CAD build for the part. Positions are in the model's coordinates, mm. Face numbers are marked on the shaded views. A direction names the side the tool comes from. Give positions to 0.01 mm unless a question says otherwise; leave off trailing zeros. Loops run counter-clockwise (first coordinate to the right, second up) from the corner with the lowest first, then second, coordinate; pieces in that order, holes last.
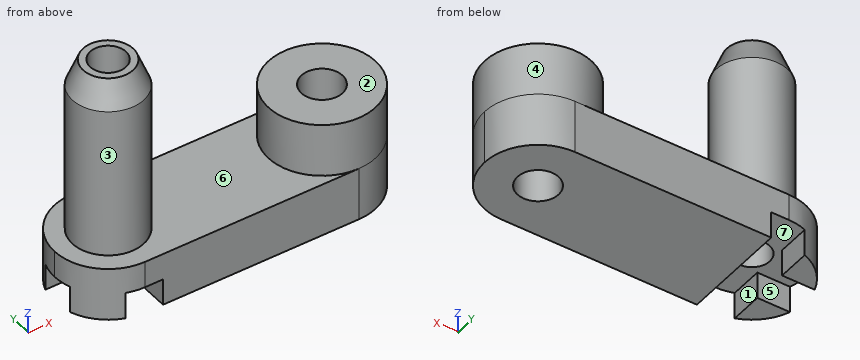
```python
from build123d import *

# Parameters (mm, degrees)
F0_W      = 18
F0_H      = 6
F1_DEPTH  = 3
F2_R      = 3
F2_R_2    = 2
F3_DEPTH  = 10
F4_R      = 1
F4_R_2    = 1.15
F5_DEPTH  = 20
F6_SIZE2  = 1.5
F6_SIZE   = 0.6
F7_W      = 11.6012076614
F7_H      = 11.8295210414
F8_DEPTH  = 7
F9_R      = 2.9999
F10_W     = 5.4413094251
F10_H     = 2
F11_DEPTH = 1.5


# Not quite as in the source:
# - a fillet or chamfer is up to 0.001 mm smaller than in the source, because OpenCascade refuses the exact size


with BuildPart() as f1:
    # F0 (on Top) → F1 (new body)
    with BuildSketch(Plane.XY):
        with Locations((1.8924829921, 0)):
            Rectangle(F0_W, F0_H)
    extrude(amount=F1_DEPTH)

    # F2 (on face) → F3 (join)
    with BuildSketch(Plane.XY.offset(3)):
        with Locations((7.8924829921, 0)):
            Circle(F2_R)
        with Locations((-4.1075170079, 0)):
            Circle(F2_R_2)
    extrude(amount=F3_DEPTH)

    # F4 (on face) → F5 (cut)
    with BuildSketch(Plane.XY.offset(13)):
        with Locations((-4.1075170079, 0)):
            Circle(F4_R)
        with Locations((7.8924829921, 0)):
            Circle(F4_R_2)
    extrude(amount=-F5_DEPTH, mode=Mode.SUBTRACT)

    # F6
    f6_edges = [f1.edges().sort_by_distance(p)[0] for p in [
        (-6.107517, 0, 13),
    ]]
    f6_side = f1.faces().sort_by_distance((-6.050948, 0, 13))[0]
    chamfer(f6_edges, length=F6_SIZE, length2=F6_SIZE2, reference=f6_side)

    # F7 (on face) → F8 (cut)
    with BuildSketch(Plane.XY.offset(13)):
        with Locations((7.5882198871, -0.5373002496)):
            Rectangle(F7_W, F7_H)
    extrude(amount=-F8_DEPTH, mode=Mode.SUBTRACT)

    # F9 (radius 3 in the source; OpenCascade refuses exactly that, so slightly less here)
    f9_edges = [f1.edges().sort_by_distance(p)[0] for p in [
        (10.892483, -3, 1.5),
        (10.892483, 3, 1.5),
        (-7.107517, 3, 1.5),
        (-7.107517, -3, 1.5),
    ]]
    fillet(f9_edges, radius=F9_R)

    # F10 (on face) → F11 (cut)
    with BuildSketch(Plane(origin=(0, 0, 0), x_dir=(1, 0, 0), z_dir=(0, 0, -1))):
        Polygon((-3.1075170079, 5.622364855), (-5.1075170079, 5.622364855), (-5.1075170079, 1), (-5.1075170079, -1), (-5.1075170079, -5.5661949279), (-3.1075170079, -5.5661949279), align=None)
        with Locations((-7.8281717205, 0)):
            Rectangle(F10_W, F10_H)
    extrude(amount=-F11_DEPTH, mode=Mode.SUBTRACT)


solid = f1.part
```
1. Probe line 1 along X through (y, z) = (0.75, 4); line 2 along Z through (x, y) = (9, -1.5); line 3 along Z through (x, y) = (0, -0.5). List the from-to ranges inside material, lowest first.
Responses:
line 1: x = -5.96 to -4.77, -3.45 to -2.25, 4.99 to 7.02, 8.76 to 10.8
line 2: z = 0 to 6
line 3: z = 0 to 3
2. Pull direction Y, two halves, no side cores. Call the marked faces 4, 5, 6 and 7: released by +Y, released by -Y, zero draft, split by the parting line, or undercut.
Responses:
face 4: split by the parting line
face 5: undercut
face 6: zero draft
face 7: undercut
3. Drop flat-ended pins along their axis: pin 1 (1.6 mm diameter, centred on y = 0, z = 0.5, fed in from -X); pin 2 (1.8 mm diameter, centred on x = 0.5, y = -1.5, fed in from +Z); pin 3 (1.5 mm diameter, centred on x = 9.5, y = -1.5, fed in from +Z); pin 4 (3 mm diameter, centred on x = -4.5, y = 0.5, fed in from +Z). Give the stop position or say it passes through.
Responses:
pin 1: stops at x = -3.11
pin 2: stops at z = 3
pin 3: stops at z = 6
pin 4: stops at z = 13
4. Tool access for the marked faces 1, 2 and 3: list every direction of +Z, -Z, +X, -X, +Y, -Y with a clear straight run to the whole face (end or side of a thin tool).
Responses:
face 1: -Z, +Y, -Y
face 2: +Z, +X, +Y, -Y
face 3: +Z
5. Saw through at D-D, the plane x = 4.5. List the corners of the cut face in (y, z), and give its area (3 significant figures).
Responses:
outline: (-3, 0) - (3, 0) - (3, 3) - (-3, 3) - close
area: 18.0 mm2
6. Saw through at B-B, the plane z = 5.25. List the corners of the cut face in (x, y), and give its area (3 significant figures).
Responses:
outline: circle Ø4 at (-4.11, 0); circle Ø6 at (7.89, 0); hole circle Ø2 at (-4.11, 0); hole circle Ø2.3 at (7.89, 0)
area: 33.5 mm2
7. Saw through at A-A, the plane z = 1.25. Count the separate pieces of the cut face and the enclosed holes in it, and give its area (3 significant figures).
Responses:
separate pieces: 3
enclosed holes: 1
area: 80.3 mm2
